Design review of the part built by this model. Coordinates are the model's own, in mm. A direction names the side the tool comes from. Coordinates: 2 decimals unless noted, no trailing zeros. Loops run counter-clockwise (first coordinate to the right, second up) from the corner with the lowest first, then second, coordinate; pieces in that order, holes last. Notation, with made-up numbers: (73, 14.5) - (129, 14.5) arc R20 ccw to (129, 32.5) - close; hole circle Ø2 at (-34.5, 68.5). An arc over 180 degrees is marked (long way). One line per question, with ' | ' between items.
from build123d import *

# Parameters (mm, degrees)
SKETCH1_W           = 62
SKETCH1_H           = 94.1
SKETCH1_R           = 1.925
BOSS_EXTRUDE1_DEPTH = 2
SKETCH2_R           = 3
CUT_EXTRUDE1_DEPTH  = 113.706743365
CUT_EXTRUDE2_DEPTH  = 113.706743365


with BuildPart() as part:
    # Sketch1 → Boss-Extrude1 (new body)
    with BuildSketch(Plane(origin=(0, 0, 0), x_dir=(1, 0, 0), z_dir=(0, 1, 0))):
        with Locations((-31, 47.05)):
            Rectangle(SKETCH1_W, SKETCH1_H)
        with Locations(Location((-56, 89.05, 0), (0, 0, 270))):
            Circle(SKETCH1_R, mode=Mode.SUBTRACT)
        with Locations(Location((-38, 89.05, 0), (0, 0, 270))):
            Circle(SKETCH1_R, mode=Mode.SUBTRACT)
        with Locations(Location((-38, 65.05, 0), (0, 0, 270))):
            Circle(SKETCH1_R, mode=Mode.SUBTRACT)
        with Locations(Location((-56, 65.05, 0), (0, 0, 270))):
            Circle(SKETCH1_R, mode=Mode.SUBTRACT)
        with Locations(Location((-56, 29.05, 0), (0, 0, 270))):
            Circle(SKETCH1_R, mode=Mode.SUBTRACT)
        with Locations(Location((-38, 29.05, 0), (0, 0, 270))):
            Circle(SKETCH1_R, mode=Mode.SUBTRACT)
        with Locations(Location((-38, 5.05, 0), (0, 0, 270))):
            Circle(SKETCH1_R, mode=Mode.SUBTRACT)
        with Locations(Location((-56, 5.05, 0), (0, 0, 270))):
            Circle(SKETCH1_R, mode=Mode.SUBTRACT)
        with Locations(Location((-24, 89.05, 0), (0, 0, 270))):
            Circle(SKETCH1_R, mode=Mode.SUBTRACT)
        with Locations(Location((-6, 89.05, 0), (0, 0, 270))):
            Circle(SKETCH1_R, mode=Mode.SUBTRACT)
        with Locations(Location((-6, 65.05, 0), (0, 0, 270))):
            Circle(SKETCH1_R, mode=Mode.SUBTRACT)
        with Locations(Location((-24, 65.05, 0), (0, 0, 270))):
            Circle(SKETCH1_R, mode=Mode.SUBTRACT)
    extrude(amount=BOSS_EXTRUDE1_DEPTH)

    # Sketch2 → Cut-Extrude1 (cut, through all)
    with BuildSketch(Plane(origin=(0, 2, 0), x_dir=(1, 0, 0), z_dir=(0, 1, 0))):
        with Locations(Location((-31, 47.05, 0), (0, 0, 270))):
            Circle(SKETCH2_R)
    extrude(amount=-CUT_EXTRUDE1_DEPTH, mode=Mode.SUBTRACT)

    # Sketch4 → Cut-Extrude2 (cut, through all)
    with BuildSketch(Plane(origin=(0, 2, 0), x_dir=(1, 0, 0), z_dir=(0, 1, 0))):
        Polygon((0, 60), (-25, 60), (-25, 0), (0, 0), (0, 33.776627829), align=None)
    extrude(amount=-CUT_EXTRUDE2_DEPTH, mode=Mode.SUBTRACT)


solid = part.part
Q1. For pin 1 (0.6 mm diameter, centred on x = -14.5, y = 0.5, fed in from +Z), flat-tipped, find the tip position at first contact; note if it passes through.
Returned:
pin 1: stops at z = -60
Q2. Take a section at B-B (z = -89.05). Give the boundary of the cut face in (x, y) (3 decimals).
Returned:
outline: (-62, 0) - (-57.925, 0) - (-57.925, 2) - (-62, 2) - close; (-54.075, 0) - (-39.925, 0) - (-39.925, 2) - (-54.075, 2) - close; (-36.075, 0) - (-25.925, 0) - (-25.925, 2) - (-36.075, 2) - close; (-22.075, 0) - (-7.925, 0) - (-7.925, 2) - (-22.075, 2) - close; (-4.075, 0) - (0, 0) - (0, 2) - (-4.075, 2) - close
Q3. Take a section at D-D (z = -47.05). Give the boundary of the cut face in (x, y).
Returned:
outline: (-62, 0) - (-34, 0) - (-34, 2) - (-62, 2) - close; (-28, 0) - (-25, 0) - (-25, 2) - (-28, 2) - close
Q4. Take a section at C-C (x = -31). Give the boundary of the cut face in (y, z).
Returned:
outline: (0, -94.1) - (2, -94.1) - (2, -50.05) - (0, -50.05) - close; (0, -44.05) - (2, -44.05) - (2, 0) - (0, 0) - close
Q5. Draft analysis for pull direction Z (two halves, no side actions). For faces 3 (the flat face through (-12, 1, -60)), 4 (the cylindrical face through (-38.737, 0.986, -63.272)), 5 (the flat face through (-38, 0, -58)), state which applies: +Z half, -Z half, draft (parallel to the pull), parting line (faces both ways), or undercut.
Returned:
face 3: +Z half | face 4: undercut | face 5: draft
Q6. To check wall thickness, follow line 1 along X through (y, z) = (1.5, -89.05) (3 decimals); line 2 along X through (y, z) = (1.75, -90); line 3 along X through (y, z) = (0.9, -30.5). State the ranges of each line that lie inside material, in increasing order.
Returned:
line 1: x = -62 to -57.925, -54.075 to -39.925, -36.075 to -25.925, -22.075 to -7.925, -4.075 to 0 | line 2: x = -62 to -57.67, -54.33 to -39.67, -36.33 to -25.67, -22.33 to -7.67, -4.33 to 0 | line 3: x = -62 to -57.27, -54.73 to -39.27, -36.73 to -25
Q7. Tool access review of faces 1 (the flat face through (-25, 1, -30)), 2 (the cylindrical face through (-56.737, 0.986, -63.272)): name each direction out of +Z, -Z, +X, -X, +Y, -Y from which nothing blocks a thin tool from reaching the whole face with its end or side.
Returned:
face 1: +Z, +X, +Y, -Y | face 2: +Y, -Y
Q8. Take a section at A-A (x = -6). Give the boundary of the cut face in (y, z) (3 decimals).
Returned:
outline: (0, -94.1) - (2, -94.1) - (2, -90.975) - (0, -90.975) - close; (0, -87.125) - (2, -87.125) - (2, -66.975) - (0, -66.975) - close; (0, -63.125) - (2, -63.125) - (2, -60) - (0, -60) - close
